For this review, take the finished solid that the model builds, in its own axes (mm). Face numbers are marked on the shaded views. Round coordinates to 2 decimals unless told otherwise and drop trailing zeros. Write each loop counter-clockwise with the first axis right and the second up, starting at its lowest first coordinate (ties: lowest second). Pieces come first, ordered by that corner, then holes. Notation, with made-up numbers: M 66.5,34 L 88.5,34 A30 ccw 88.5,56 Z; hole C 82.25,-13.75 d9. An arc over 180 degrees is marked long. Answer in a Markdown table with one row per item.
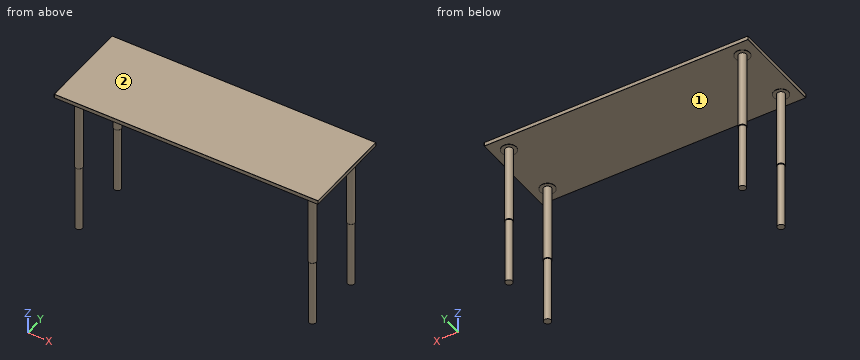
```python
from build123d import *

# Parameters (mm, degrees)
F0_W      = 1879.6
F0_H      = 650.875
F1_DEPTH  = 28.2
F2_R      = 1
F3_R      = 52.1
F4_DEPTH  = 2.62
F5_R      = 27.6
F6_DEPTH  = 558.8
F8_R      = 24.95
F9_DEPTH  = 473.075
F6_FACE_R = 27.6
F9_FACE_R = 24.95


with BuildPart() as f1:
    # F0 (on Top) → F1 (new body)
    with BuildSketch(Plane.XY):
        Rectangle(F0_W, F0_H)
    extrude(amount=F1_DEPTH)

    # F2
    f2_edges = [f1.edges().sort_by_distance(p)[0] for p in [
        (0, -325.4375, 28.2),
        (0, -325.4375, 0),
        (-939.8, 0, 28.2),
        (0, 325.4375, 28.2),
        (939.8, 0, 28.2),
        (939.8, 0, 0),
        (0, 325.4375, 0),
        (-939.8, 0, 0),
        (-939.8, -325.4375, 14.1),
        (-939.8, 325.4375, 14.1),
        (939.8, 325.4375, 14.1),
        (939.8, -325.4375, 14.1),
    ]]
    fillet(f2_edges, radius=F2_R)

    # F3 (on face) → F4 (join)
    with BuildSketch(Plane(origin=(0, 0, 0), x_dir=(1, 0, 0), z_dir=(0, 0, -1))):
        with Locations((-831.7, 217.3375)):
            Circle(F3_R)
    extrude(amount=F4_DEPTH)

    # F5 (on face) → F6 (join)
    with BuildSketch(Plane(origin=(0, 0, -2.62), x_dir=(1, 0, 0), z_dir=(0, 0, -1))):
        with Locations((-831.7, 217.3375)):
            Circle(F5_R)
    extrude(amount=F6_DEPTH)



with BuildPart() as f9:
    # F8 (on offset) → F9 (new body)
    with BuildSketch(Plane(origin=(0, 0, -564.85), x_dir=(1, 0, 0), z_dir=(0, 0, -1))):
        with Locations((-831.7, 217.3375)):
            Circle(F8_R)
    extrude(amount=F9_DEPTH)


with BuildPart() as f1_1:
    add(f1.part)

    add(f9.part)  # F10 merges F9
    # F6_face (on face) → F10 section 0
    with BuildSketch(Plane(origin=(-831.7, -217.3375, -561.42), x_dir=(1, 0, 0), z_dir=(0, 0, -1))):
        Circle(F6_FACE_R)
    # F9_face (on face) → F10 section 1
    with BuildSketch(Plane(origin=(-831.7, -217.3375, -564.85), x_dir=(1, 0, 0), z_dir=(0, 0, 1))):
        Circle(F9_FACE_R)
    loft()

    # F11: F1 across plane


with BuildPart() as f1_2:
    add(f1_1.part)
    add(f1_1.part.mirror(Plane.XZ))

    # F12: F1 across plane


with BuildPart() as f1_3:
    add(f1_2.part)
    add(f1_2.part.mirror(Plane.YZ))


solid = f1_3.part
```
Q1. Take a section at B-B (y = 24.5). State the section outline as (x, z) points.
Found:
| item | result |
|---|---|
| outline | M -939.8,1 A1 ccw -938.8,0 L 938.8,0 A1 ccw 939.8,1 L 939.8,27.2 A1 ccw 938.8,28.2 L -938.8,28.2 A1 ccw -939.8,27.2 Z |
Q2. Mouldability with a two-part tool opening along X and no side actions: class the marked faces 1 and 2 as +X half, -X half, draft (parallel to the pull), parting line (faces both ways), or undercut.
Found:
| item | result |
|---|---|
| face 1 | undercut |
| face 2 | draft |
Q3. Take a section at C-C (z = -291). State the section outline as (x, y) points.
Found:
| item | result |
|---|---|
| outline | C -831.7,-217.34 d55.2; C -831.7,217.34 d55.2; C 831.7,-217.34 d55.2; C 831.7,217.34 d55.2 |
Q4. For probe 1 along Y at (x, z) = (844, -148); probe 2 along Z at (x, y) = (330, -175); probe 3 along Y at (x, z) = (-831.5, -711), list the stretches that pass through material, from the lowest coordinate up.
Found:
| item | result |
|---|---|
| probe 1 | -242.05 to -192.63, 192.63 to 242.05 |
| probe 2 | 0 to 28.2 |
| probe 3 | -242.29 to -192.39, 192.39 to 242.29 |
Q5. Take a section at A-A (x = 244.5). State the section outline as (y, z) points, then the cut area to 3 significant figures.
Found:
| item | result |
|---|---|
| outline | M -325.44,1 A1 ccw -324.44,0 L 324.44,0 A1 ccw 325.44,1 L 325.44,27.2 A1 ccw 324.44,28.2 L -324.44,28.2 A1 ccw -325.44,27.2 Z |
| area | 18,400 mm² |
